```python
from build123d import *

# Parameters (mm, degrees)
SKETCH1_W           = 6
SKETCH1_H           = 6
BOSS_EXTRUDE1_DEPTH = 3
HOLE1_D             = 4
HOLE1_DEPTH         = 3
HOLE1_CBORE_D       = 5
HOLE1_CBORE_DEPTH   = 0.8
HOLE1_TIP           = 1.201721238
CUT_EXTRUDE1_START  = -0.8
SKETCH4_R           = 2.5
CUT_EXTRUDE1_DEPTH  = 0.8
LPATTERN1_COUNT     = 3
LPATTERN1_PITCH     = 6
LPATTERN1_2_COUNT   = 7
LPATTERN1_2_PITCH   = 6
FILLET5_R           = 3


with BuildPart() as part:
    # Sketch1 → Boss-Extrude1 (new body)
    with BuildSketch(Plane.XY):
        with Locations((-3, 3)):
            Rectangle(SKETCH1_W, SKETCH1_H)
    extrude(amount=BOSS_EXTRUDE1_DEPTH)

    # Hole1
    with Locations(Plane.XY.offset(3)):
        with Locations((-3, 3)):
            CounterBoreHole(HOLE1_D / 2, HOLE1_CBORE_D / 2, HOLE1_CBORE_DEPTH, depth=HOLE1_DEPTH)
            with Locations((0, 0, -(HOLE1_DEPTH + HOLE1_TIP / 2))):  # 118° drill point
                Cone(0, HOLE1_D / 2, HOLE1_TIP, mode=Mode.SUBTRACT)

    # Sketch4 → Cut-Extrude1 (cut)
    with BuildSketch(Plane(origin=(0, 0, 0), x_dir=(-1, 0, 0), z_dir=(0, 0, -1)).offset(CUT_EXTRUDE1_START)):
        with Locations(Location((3, 3, 0), (0, 0, 180))):
            Circle(SKETCH4_R)
    extrude(amount=CUT_EXTRUDE1_DEPTH, mode=Mode.SUBTRACT)


with BuildPart() as lpattern1_1:
    # LPattern1: pattern copy
    add(part.part.moved(Location(Vector(0, 1, 0) * (1 * LPATTERN1_PITCH))))


with BuildPart() as lpattern1_2:
    # LPattern1: pattern copy
    add(part.part.moved(Location(Vector(0, 1, 0) * (2 * LPATTERN1_PITCH))))


with BuildPart() as lpattern1_2_1:
    # LPattern1 2: pattern copy
    add(part.part.moved(Location(Vector(1, 0, 0) * (1 * LPATTERN1_2_PITCH))))


with BuildPart() as lpattern1_2_2:
    # LPattern1 2: pattern copy
    add(part.part.moved(Location(Vector(1, 0, 0) * (2 * LPATTERN1_2_PITCH))))


with BuildPart() as lpattern1_2_3:
    # LPattern1 2: pattern copy
    add(part.part.moved(Location(Vector(1, 0, 0) * (3 * LPATTERN1_2_PITCH))))


with BuildPart() as lpattern1_2_4:
    # LPattern1 2: pattern copy
    add(part.part.moved(Location(Vector(1, 0, 0) * (4 * LPATTERN1_2_PITCH))))


with BuildPart() as lpattern1_2_5:
    # LPattern1 2: pattern copy
    add(part.part.moved(Location(Vector(1, 0, 0) * (5 * LPATTERN1_2_PITCH))))


with BuildPart() as lpattern1_2_6:
    # LPattern1 2: pattern copy
    add(part.part.moved(Location(Vector(1, 0, 0) * (6 * LPATTERN1_2_PITCH))))


with BuildPart() as lpattern1_2_7:
    # LPattern1 2: pattern copy
    add(lpattern1_1.part.moved(Location(Vector(1, 0, 0) * (1 * LPATTERN1_2_PITCH))))


with BuildPart() as lpattern1_2_8:
    # LPattern1 2: pattern copy
    add(lpattern1_1.part.moved(Location(Vector(1, 0, 0) * (2 * LPATTERN1_2_PITCH))))


with BuildPart() as lpattern1_2_9:
    # LPattern1 2: pattern copy
    add(lpattern1_1.part.moved(Location(Vector(1, 0, 0) * (3 * LPATTERN1_2_PITCH))))


with BuildPart() as lpattern1_2_10:
    # LPattern1 2: pattern copy
    add(lpattern1_1.part.moved(Location(Vector(1, 0, 0) * (4 * LPATTERN1_2_PITCH))))


with BuildPart() as lpattern1_2_11:
    # LPattern1 2: pattern copy
    add(lpattern1_1.part.moved(Location(Vector(1, 0, 0) * (5 * LPATTERN1_2_PITCH))))


with BuildPart() as lpattern1_2_12:
    # LPattern1 2: pattern copy
    add(lpattern1_1.part.moved(Location(Vector(1, 0, 0) * (6 * LPATTERN1_2_PITCH))))


with BuildPart() as lpattern1_2_13:
    # LPattern1 2: pattern copy
    add(lpattern1_2.part.moved(Location(Vector(1, 0, 0) * (1 * LPATTERN1_2_PITCH))))


with BuildPart() as lpattern1_2_14:
    # LPattern1 2: pattern copy
    add(lpattern1_2.part.moved(Location(Vector(1, 0, 0) * (2 * LPATTERN1_2_PITCH))))


with BuildPart() as lpattern1_2_15:
    # LPattern1 2: pattern copy
    add(lpattern1_2.part.moved(Location(Vector(1, 0, 0) * (3 * LPATTERN1_2_PITCH))))


with BuildPart() as lpattern1_2_16:
    # LPattern1 2: pattern copy
    add(lpattern1_2.part.moved(Location(Vector(1, 0, 0) * (4 * LPATTERN1_2_PITCH))))


with BuildPart() as lpattern1_2_17:
    # LPattern1 2: pattern copy
    add(lpattern1_2.part.moved(Location(Vector(1, 0, 0) * (5 * LPATTERN1_2_PITCH))))


with BuildPart() as lpattern1_2_18:
    # LPattern1 2: pattern copy
    add(lpattern1_2.part.moved(Location(Vector(1, 0, 0) * (6 * LPATTERN1_2_PITCH))))


with BuildPart() as part_1:
    add(part.part)

    # Combine3: union LPattern1_1, LPattern1_2, LPattern1 2_1, LPattern1 2_7, LPattern1 2_13, LPattern1 2_2, LPattern1 2_8, LPattern1 2_14, LPattern1 2_3, LPattern1 2_9, LPattern1 2_15, LPattern1 2_4, LPattern1 2_10, LPattern1 2_16, LPattern1 2_5, LPattern1 2_11, LPattern1 2_17, LPattern1 2_6, LPattern1 2_12, LPattern1 2_18
    add(lpattern1_1.part)
    add(lpattern1_2.part)
    add(lpattern1_2_1.part)
    add(lpattern1_2_7.part)
    add(lpattern1_2_13.part)
    add(lpattern1_2_2.part)
    add(lpattern1_2_8.part)
    add(lpattern1_2_14.part)
    add(lpattern1_2_3.part)
    add(lpattern1_2_9.part)
    add(lpattern1_2_15.part)
    add(lpattern1_2_4.part)
    add(lpattern1_2_10.part)
    add(lpattern1_2_16.part)
    add(lpattern1_2_5.part)
    add(lpattern1_2_11.part)
    add(lpattern1_2_17.part)
    add(lpattern1_2_6.part)
    add(lpattern1_2_12.part)
    add(lpattern1_2_18.part)

    # Fillet5
    fillet5_edges = [part_1.edges().sort_by_distance(p)[0] for p in [
        (-6, 18, 1.5),
        (36, 18, 1.5),
        (36, 0, 1.5),
        (-6, 0, 1.5),
    ]]
    fillet(fillet5_edges, radius=FILLET5_R)


solid = part_1.part
```
Input: part model. Units: mm. Frame: model coordinates. A direction names the side the tool comes from. Round coordinates to 2 decimals unless told otherwise and drop trailing zeros. One line per item, written item: value.
(1) Set-up query: faces 1 (the face through (8.46, 12.56, 2.61)), 2 (the face through (3, 1, 1)), 3 (the face through (-3.54, 11.44, 0.41)). Return all of +Z, -Z, +X, -X, +Y, -Y with unobstructed straight access to the full face (end or side cutting, diameter ignored); none if empty.
Geometry check:
face 1: +Z
face 2: +Z, -Z
face 3: -Z
(2) Pin query (flat end, axial travel): pin 1 (6.5 mm diameter, centred on x = -3, y = 15, fed in from +Z); pin 2 (2.5 mm diameter, centred on x = -3, y = 15, fed in from +Z). Return the tip coordinate at first contact, or that it passes through.
Geometry check:
pin 1: z = 3
pin 2: through
(3) Material intervals for line 1 (Y direction, x = -3, z = 2.7); line 2 (Y direction, x = 3, z = 1.85), sorted ascending. Write a range as [from, to].
Geometry check:
line 1: [0, 0.5], [5.5, 6.5], [11.5, 12.5], [17.5, 18]
line 2: [0, 1], [5, 7], [11, 13], [17, 18]
(4) Section A-A (z = 1.3). Give the number of separate pieces and of enclosed holes in the cut face, plus the area to 3 significant figures.
Geometry check:
separate pieces: 1
enclosed holes: 21
area: 484 mm2
(5) Mould query, pull axis Y, two halves, no side actions, for faces 4 (the face through (8.46, 17.44, 0.41)), 5 (the face through (12.5, 15.1, 2.6)). Classes: pulls with the +Y half, pulls with the -Y half, needs draft (parallel to the pull), parting line crosses it, or undercut.
Geometry check:
face 4: undercut
face 5: undercut
